The model under review builds one solid part; all positions refer to its coordinate system, in mm. A direction names the side the tool comes from. Coordinates: 2 decimals unless noted, no trailing zeros. Order: outer loops, then holes, each group sorted by start corner. A loop starts at its lowest first (then second) coordinate and runs counter-clockwise, first axis right, second up. Notation, with made-up numbers: (63.25, 20.5) -> (79.25, 20.5) arc R27 cw to (79.25, 46.5) -> close; hole circle Ø2 at (-14, 55). An arc over 180 degrees is marked (long way). Use one line per item in the form item = value.
Autodesk Inventor part; units mm, degrees
ref_plane "YZ Plane" through (0, 0, 0) normal (1, 0, 0) x (0, 1, 0)
ref_plane "XZ Plane" through (0, 0, 0) normal (0, 1, 0) x (-1, 0, 0)
ref_plane "XY Plane" through (0, 0, 0) normal (0, 0, 1) x (1, 0, 0)
sketch "Sketch1" plane through (0, 0, 0) normal (0, 0, 1) x (1, 0, 0)
  line L0 (11.176, -9.652) -> (11.176, 9.652)
  arc A0 (9.652, -11.176) -> (11.176, -9.652) centre (9.652, -9.652) ccw
  line L1 (-9.652, -11.176) -> (9.652, -11.176)
  arc A1 (-11.176, -9.652) -> (-9.652, -11.176) centre (-9.652, -9.652) ccw
  line L2 (-11.176, 9.652) -> (-11.176, -9.652)
  arc A2 (-9.652, 11.176) -> (-11.176, 9.652) centre (-9.652, 9.652) ccw
  line L3 (9.652, 11.176) -> (-9.652, 11.176)
  arc A3 (11.176, 9.652) -> (9.652, 11.176) centre (9.652, 9.652) ccw
  arc A4 (12.7, -4.064) -> (13.462, -4.826) centre (13.462, -4.064) ccw
  line L4 (12.7, -4.064) -> (12.7, 10.5918)
  arc A5 (12.7, 10.5918) -> (10.5918, 12.7) centre (10.5918, 10.5918) ccw
  line L5 (10.5918, 12.7) -> (-10.5918, 12.7)
  arc A6 (-10.5918, 12.7) -> (-12.7, 10.5918) centre (-10.5918, 10.5918) ccw
  line L6 (-12.7, 10.5918) -> (-12.7, -4.064)
  arc A7 (-13.462, -4.826) -> (-12.7, -4.064) centre (-13.462, -4.064) ccw
  line L7 (-13.462, -4.826) -> (-24.638, -4.826)
  arc A8 (-24.638, -4.826) -> (-24.638, -6.35) centre (-24.638, -5.588) ccw
  line L8 (-24.638, -6.35) -> (-13.462, -6.35)
  arc A9 (-12.7, -7.112) -> (-13.462, -6.35) centre (-13.462, -7.112) ccw
  line L9 (-12.7, -7.112) -> (-12.7, -10.5918)
  arc A10 (-12.7, -10.5918) -> (-10.5918, -12.7) centre (-10.5918, -10.5918) ccw
  line L10 (-10.5918, -12.7) -> (10.5918, -12.7)
  arc A11 (10.5918, -12.7) -> (12.7, -10.5918) centre (10.5918, -10.5918) ccw
  line L11 (12.7, -10.5918) -> (12.7, -7.112)
  arc A12 (13.462, -6.35) -> (12.7, -7.112) centre (13.462, -7.112) ccw
  line L12 (13.462, -6.35) -> (24.638, -6.35)
  arc A13 (24.638, -6.35) -> (24.638, -4.826) centre (24.638, -5.588) ccw
  line L13 (24.638, -4.826) -> (13.462, -4.826)
  point P0 (0, 0)
extrude "Extrusion1" add sketch "Sketch1" against normal blind 304.8
properties part number "9015"
Item 1: We need section C-C (z = -248). Write out the cut boundary in (x, y).
Results found:
outline = (-24.64, -6.35) -> (-13.46, -6.35) arc R0.76 cw to (-12.7, -7.11) -> (-12.7, -10.59) arc R2.11 ccw to (-10.59, -12.7) -> (10.59, -12.7) arc R2.11 ccw to (12.7, -10.59) -> (12.7, -7.11) arc R0.76 cw to (13.46, -6.35) -> (24.64, -6.35) arc R0.76 ccw to (24.64, -4.83) -> (13.46, -4.83) arc R0.76 cw to (12.7, -4.06) -> (12.7, 10.59) arc R2.11 ccw to (10.59, 12.7) -> (-10.59, 12.7) arc R2.11 ccw to (-12.7, 10.59) -> (-12.7, -4.06) arc R0.76 cw to (-13.46, -4.83) -> (-24.64, -4.83) arc R0.76 ccw to start; hole (-11.18, -9.65) arc R1.52 ccw to (-9.65, -11.18) -> (9.65, -11.18) arc R1.52 ccw to (11.18, -9.65) -> (11.18, 9.65) arc R1.52 ccw to (9.65, 11.18) -> (-9.65, 11.18) arc R1.52 ccw to (-11.18, 9.65) -> close
Item 2: Draft analysis for pull direction X (two halves, no side actions). For faces 6 (the face through (0, 11.176, -150)), 7 (the face through (0, -12.7, -150)), 8 (the face through (-12.7, 3, -150)), 9 (the face through (0, -11.176, -150)), state which applies: released by +X, released by -X, zero draft, split by the parting line, or undercut.
Results found:
face_6 = undercut
face_7 = zero draft
face_8 = released by -X
face_9 = undercut
Item 3: We need section D-D (x = 16.5). Write out the cut boundary in (y, z), plus the area to 3 significant figures.
Results found:
outline = (-6.35, -304.8) -> (-4.83, -304.8) -> (-4.83, 0) -> (-6.35, 0) -> close
area = 465 mm²
Item 4: Clearance check with flat-ended pins moving along their axes: pin 1 (12 mm diameter, centred on y = 3, z = -251.5, fed in from +X); pin 2 (5.5 mm diameter, centred on x = 19.5, z = -201, fed in from -Y); pin 3 (5.5 mm diameter, centred on x = 16.5, z = -152.5, fed in from +Y). State where each tip first meets the part, or that it passes through.
Results found:
pin_1 = 12.7
pin_2 = -6.35
pin_3 = -4.83
Item 5: Tool access review of faces 1 (the face through (19, -4.826, -150)), 2 (the face through (-19, -6.35, -150)), 3 (the face through (-19, -4.826, -150)), 4 (the face through (11.176, 0, -150)), 5 (the face through (19, -6.35, -150)): name each direction out of +Z, -Z, +X, -X, +Y, -Y from which nothing blocks a thin tool from reaching the whole face with its end or side.
Results found:
face_1 = +Z, -Z, +X, +Y
face_2 = +Z, -Z, -X, -Y
face_3 = +Z, -Z, -X, +Y
face_4 = +Z, -Z
face_5 = +Z, -Z, +X, -Y
Item 6: We need section A-A (y = -0.5). Write out the cut boundary in (x, z).
Results found:
outline = (-12.7, -304.8) -> (-11.18, -304.8) -> (-11.18, 0) -> (-12.7, 0) -> close; (11.18, -304.8) -> (12.7, -304.8) -> (12.7, 0) -> (11.18, 0) -> close
Item 7: To check wall thickness, follow L1, parallel to Y at x = -3, z = -278; L2, parallel to Y at x = 15, z = -292. State the ranges of each line that lie inside material, in increasing order. Write a range as from..to.
Results found:
L1 = -12.7..-11.18, 11.18..12.7
L2 = -6.35..-4.83
